For this review, take the finished solid that the model builds, in its own axes (mm). A direction names the side the tool comes from. Give positions to 0.01 mm unless a question says otherwise; leave off trailing zeros. Order: outer loops, then holes, each group sorted by start corner. A loop starts at its lowest first (then second) coordinate and runs counter-clockwise, first axis right, second up. Notation, with made-up numbers: (-17, 59.5) -> (19, 59.5) arc R22 ccw to (19, 90.5) -> close; hole circle Ø3 at (-17.75, 37.25). An arc over 180 degrees is marked (long way). One line per item, written item: value. Start each with the question number.
from build123d import *

# Parameters (mm, degrees)
SKETCH1_R           = 100
SKETCH1_R_2         = 26.5
BOSS_EXTRUDE1_DEPTH = 70
SKETCH2_W           = 55
SKETCH2_H           = 60


with BuildPart() as part:
    # Sketch1 → Boss-Extrude1 (new body)
    with BuildSketch(Plane.XY):
        Circle(SKETCH1_R)
        Circle(SKETCH1_R_2, mode=Mode.SUBTRACT)
    extrude(amount=BOSS_EXTRUDE1_DEPTH)

    # Sketch2 → Cut-Revolve1 (revolve, cut)
    with BuildSketch(Plane(origin=(0, 0, 0), x_dir=(1, 0, 0), z_dir=(0, 1, 0)), mode=Mode.PRIVATE) as cut_revolve1_sk:
        with Locations((-72.5, -35)):
            Rectangle(SKETCH2_W, SKETCH2_H)
    revolve(cut_revolve1_sk.sketch.rotate(Axis((0, 0, 0), (0, 0, -1)), 180), axis=Axis((0, 0, 0), (0, 0, -1)), mode=Mode.SUBTRACT)


solid = part.part
Q1. Mouldability with a two-part tool opening along Z and no side actions: class faces 3 (the cylindrical face through (14.246, 22.345, 34.51)), 4 (the flat face through (21, -21, 0)), 5 (the cylindrical face through (20.765, 39.923, 34.58)), 6 (the flat face through (21, -21, 70)) as pulls with the +Z half, pulls with the -Z half, needs draft (parallel to the pull), parting line crosses it, or undercut.
Q2. Take a section at D-D (x = 63). State the section outline as (y, z) points, and give its area (3 significant figures).
Q3. For line 1 along Z through (x, y) = (90, 28.5); line 2 along Y through (x, z) = (-1.5, 10) (3 decimals); line 3 along Y through (x, z) = (-20.5, 14.5), list the stretches that pass through material, from the lowest coordinate up.
Q4. Take a section at C-C (z = 37). State the section outline as (x, y) points, and give its area (3 significant figures).
Q5. For faces 1 (the cylindrical face through (95.38, 30.04, 2.46)), 2 (the flat face through (21, 43, 65)), list the 3-axis set-ups (+Z, -Z, +X, -X, +Y, -Y) from which the entire face can be reached by the end or side of a thin tool; tool diameter is ignored.
Q6. For pin 1 Ø6 at (x, z) = (-49, 34) entering from +Y; pin 2 Ø10 at (x, z) = (-29, 13.5) entering from +Y; pin 3 Ø2 at (x, z) = (8.5, 36.5) entering from +Y; pin 4 Ø3 at (y, z) = (-9.5, 45) entering from -X, all flat-tipped, find the tip position at first contact; note any pin that passes through.
Q7. Take a section at A-A (y = 0). State the section outline as (x, z) points.
Answers below:
1. face 3: needs draft
1. face 4: pulls with the -Z half
1. face 5: undercut
1. face 6: pulls with the +Z half
2. outline: (-77.66, 0) -> (77.66, 0) -> (77.66, 5) -> (-77.66, 5) -> close; (-77.66, 65) -> (77.66, 65) -> (77.66, 70) -> (-77.66, 70) -> close
2. area: 1,550 mm²
3. line 1: z = 0 to 5, 65 to 70
3. line 2: y = -44.975 to -26.458, 26.458 to 44.975
3. line 3: y = -40.06 to -16.79, 16.79 to 40.06
4. outline: circle Ø90 at (0, 0); hole circle Ø53 at (0, 0)
4. area: 4,160 mm²
5. face 1: +Z, -Z
5. face 2: none
6. pin 1: passes through
6. pin 2: stops at y = 38.07
6. pin 3: stops at y = 44.37
6. pin 4: stops at x = -44.28
7. outline: (-100, 0) -> (-26.5, 0) -> (-26.5, 70) -> (-100, 70) -> (-100, 65) -> (-45, 65) -> (-45, 5) -> (-100, 5) -> close; (26.5, 0) -> (100, 0) -> (100, 5) -> (45, 5) -> (45, 65) -> (100, 65) -> (100, 70) -> (26.5, 70) -> close
